Can you work these out from the model? Positions are in its coordinate system, mm. Face numbers are marked on the shaded views. A direction names the side the tool comes from. Round coordinates to 2 decimals unless told otherwise and drop trailing zeros. Loops run counter-clockwise (first coordinate to the right, second up) from the corner with the lowest first, then second, coordinate; pieces in that order, holes last.
from build123d import *

# Parameters (mm, degrees)
SKICA1_W                = 20
SKICA1_H                = 20
SKICA1_R                = 4.25
P_IDAT_VYSUNUT_M1_DEPTH = 2
P_IDAT_START            = -2
SKICA2_W                = 20
SKICA2_H                = 3
P_IDAT_VYSUNUT_M2_DEPTH = 15
P_IDAT_VYSUNUT_M3_DEPTH = 2
ZAOBLIT1_R              = 2
ZAOBLIT2_R              = 2


with BuildPart() as part:
    # Skica1 → Přidat vysunutím1 (new body)
    with BuildSketch(Plane.XY):
        with Locations((0, -3)):
            Rectangle(SKICA1_W, SKICA1_H)
        Circle(SKICA1_R, mode=Mode.SUBTRACT)
    extrude(amount=-P_IDAT_VYSUNUT_M1_DEPTH)

    # Skica2 → Přidat vysunutím2 (add)
    with BuildSketch(Plane(origin=(0, 0, -2), x_dir=(-1, 0, 0), z_dir=(0, 0, -1)).offset(P_IDAT_START)):
        with Locations((0, -11.5)):
            Rectangle(SKICA2_W, SKICA2_H)
    extrude(amount=P_IDAT_VYSUNUT_M2_DEPTH)

    # Skica3 → Přidat vysunutím3 (add)
    with BuildSketch(Plane.ZY.offset(10)):
        Polygon((-2, -10), (-7, -10), (-2, -5), align=None)
    p_idat_vysunut_m3 = extrude(amount=-P_IDAT_VYSUNUT_M3_DEPTH)

    # Zrcadlit1: Přidat vysunutím3 across plane
    add(p_idat_vysunut_m3.mirror(Plane(origin=(0, 0, 0), x_dir=(0, 0, 1), z_dir=(1, 0, 0))))

    # Zaoblit1
    zaoblit1_edges = [part.edges().sort_by_distance(p)[0] for p in [
        (-10, 7, -1),
        (10, 7, -1),
    ]]
    fillet(zaoblit1_edges, radius=ZAOBLIT1_R)

    # Zaoblit2
    zaoblit2_edges = [part.edges().sort_by_distance(p)[0] for p in [
        (-10, -11.5, -15),
        (10, -11.5, -15),
    ]]
    fillet(zaoblit2_edges, radius=ZAOBLIT2_R)


solid = part.part
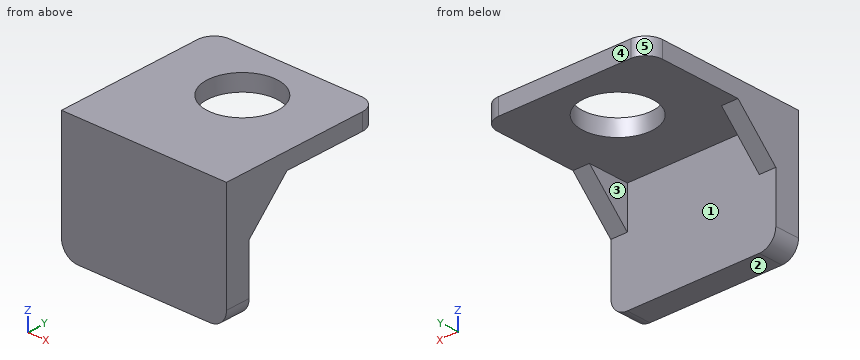
(1) If we section it at A-A, the plane x = 0: List the corners of the cut face in (y, z) for me, then the cut area to 3 significant figures.
Worked answers:
outline: (-13, -15) - (-10, -15) - (-10, -2) - (-4.25, -2) - (-4.25, 0) - (-13, 0) - close; (4.25, -2) - (7, -2) - (7, 0) - (4.25, 0) - close
area: 62.0 mm2
(2) Will these pins go through, and if not, where does the flat tip stop? P1, Ø6, axis at x = -1, z = -6, coming from the +Y side; P2, Ø4, axis at y = 1, z = -5, coming from the -X side; P3, Ø10, axis at x = 0, y = 0, coming from the -Z side.
Worked answers:
P1: stops at y = -10
P2: passes through
P3: stops at z = -2
(3) If I drill on line 1 (Y direction, x = 0, z = -1.45); line 2 (Z direction, x = -6, y = 0.5); line 3 (Y direction, x = 2.5, z = -11), over which ranges is the centre line in solid material (lowest first)?
Worked answers:
line 1: y = -13 to -4.25, 4.25 to 7
line 2: z = -2 to 0
line 3: y = -13 to -10
(4) If we section it at B-B, the plane z = -1.5: List the corners of the cut face in (x, y) for me.
Worked answers:
outline: (-10, -13) - (10, -13) - (10, 5) arc R2 ccw to (8, 7) - (-8, 7) arc R2 ccw to (-10, 5) - close; hole circle Ø8.5 at (0, 0)
(5) If we section it at C-C, the plane y = 0: List the corners of the cut face in (x, z) for me, then the cut area to 3 significant figures.
Worked answers:
outline: (-10, -2) - (-4.25, -2) - (-4.25, 0) - (-10, 0) - close; (4.25, -2) - (10, -2) - (10, 0) - (4.25, 0) - close
area: 23.0 mm2
(6) If we mould it in two halves opening along X, with no side actions, what happens to the marked faces 3, 4 and 5? For each: released by +X, released by -X, zero draft, split by the parting line, or undercut.
Worked answers:
face 3: undercut
face 4: zero draft
face 5: released by -X
(7) For the marked faces 1 and 2, which set-ups out of +Z, -Z, +X, -X, +Y, -Y let a thin tool reach every point of the face, with its end or its side?
Worked answers:
face 1: -Z, +Y
face 2: -Z, +X, -X, +Y, -Y
(8) If we section it at D-D, the plane y = -6.75: List the corners of the cut face in (x, z) for me.
Worked answers:
outline: (-10, -3.75) - (-8, -3.75) - (-8, -2) - (8, -2) - (8, -3.75) - (10, -3.75) - (10, 0) - (-10, 0) - close
